```python
from build123d import *

# Parameters (mm, degrees)
BOSS_EXTRUDE1_DEPTH = 6
SKETCH2_R           = 5.25
CUT_EXTRUDE1_DEPTH  = 88
SKETCH2_2_R         = 5.25
BOSS_EXTRUDE2_DEPTH = 12
BOSS_EXTRUDE3_START = -24.75
SKETCH2_3_R         = 5.25
BOSS_EXTRUDE3_DEPTH = 10.25
SKETCH3_W           = 4
SKETCH3_H           = 8.859259966
BOSS_EXTRUDE4_DEPTH = 3
BOSS_EXTRUDE5_DEPTH = 3.5
CUT_EXTRUDE2_DEPTH  = 84.5
SKETCH14_W          = 24
SKETCH14_H          = 3
BOSS_EXTRUDE9_DEPTH = 0.5
BOSS_EXTRUDE7_DEPTH = 3.5
SKETCH12_W          = 11
SKETCH12_H          = 7.5
BOSS_EXTRUDE8_DEPTH = 8
SKETCH13_W          = 3
SKETCH13_H          = 5.5
CUT_EXTRUDE5_DEPTH  = 5.5
FILLET6_R           = 4.5
HOLE1_START         = -35
HOLE1_OUTLINE_R     = 3
HOLE1_DEPTH         = 70
CUT_EXTRUDE3_DEPTH  = 84.5
CHAMFER1_SIZE       = 2
FILLET3_R           = 2
BOSS_EXTRUDE6_REACH = 58.524
SKETCH9_W           = 1.5
SKETCH9_H           = 4
FILLET4_R           = 0.75
FILLET5_R           = 6


# Read off the part's stored shape, not the designer's step: Hole1
with BuildPart() as part:
    # Sketch1 → Boss-Extrude1 (new body)
    with BuildSketch(Plane.XY):
        Polygon((-25, 0), (25, 0), (35, 7.002075382), (35, 25), (-35, 25), (-35, 7.002075382), align=None)
    extrude(amount=BOSS_EXTRUDE1_DEPTH)

    # Sketch2 → Cut-Extrude1 (cut)
    with BuildSketch(Plane(origin=(35, 0, 0), x_dir=(0, 0, -1), z_dir=(1, 0, 0))):
        with Locations((-6, 12.452075382)):
            Circle(SKETCH2_R)
    extrude(amount=-CUT_EXTRUDE1_DEPTH, mode=Mode.SUBTRACT)

    # Sketch2<2> → Boss-Extrude2 (add)
    with BuildSketch(Plane(origin=(35, 0, 0), x_dir=(0, 0, -1), z_dir=(1, 0, 0))):
        with Locations((-6, 12.452075382)):
            Circle(SKETCH2_2_R)
    boss_extrude2 = extrude(amount=-BOSS_EXTRUDE2_DEPTH)

    # Sketch2<3> → Boss-Extrude3 (add)
    with BuildSketch(Plane(origin=(35, 0, 0), x_dir=(0, 0, -1), z_dir=(1, 0, 0)).offset(BOSS_EXTRUDE3_START)):
        with Locations((-6, 12.452075382)):
            Circle(SKETCH2_3_R)
    boss_extrude3 = extrude(amount=-BOSS_EXTRUDE3_DEPTH)

    # Sketch3 → Boss-Extrude4 (add)
    with BuildSketch(Plane(origin=(0, 0, 0), x_dir=(-1, 0, 0), z_dir=(0, 0, -1))):
        with Locations((2, -11.570370017)):
            Rectangle(SKETCH3_W, SKETCH3_H)
        Polygon((0, -7.140740034), (4, -7.140740034), (9, 0), (0, 0), align=None)
    boss_extrude4 = extrude(amount=-BOSS_EXTRUDE4_DEPTH)

    # Sketch4 → Boss-Extrude5 (add)
    with BuildSketch(Plane.XY.offset(6)):
        with BuildLine():
            Line((26, 10.749226565), (26, 18.202075382))
            ThreePointArc((26, 18.202075382), (28, 20.202075382), (30, 18.202075382))
            Line((30, 18.202075382), (30, 10.749226565))
            ThreePointArc((30, 10.749226565), (28, 8.749226565), (26, 10.749226565))
        make_face()
    boss_extrude5 = extrude(amount=BOSS_EXTRUDE5_DEPTH)

    # Sketch5 → Cut-Extrude2 (cut)
    with BuildSketch(Plane(origin=(35, 0, 0), x_dir=(0, 0, -1), z_dir=(1, 0, 0))):
        Polygon((-1, 25), (-1, 24.5), (-5, 21.5), (-5, 21), (-6, 21), (-6, 25), align=None)
    extrude(amount=-CUT_EXTRUDE2_DEPTH, mode=Mode.SUBTRACT)

    # Mirror2: Boss-Extrude2, Boss-Extrude3, Boss-Extrude4, Boss-Extrude5 across plane
    add(boss_extrude2.mirror(Plane(origin=(0, 0, 3), x_dir=(0, 0, 1), z_dir=(-1, 0, 0))))
    add(boss_extrude3.mirror(Plane(origin=(0, 0, 3), x_dir=(0, 0, 1), z_dir=(-1, 0, 0))))
    add(boss_extrude4.mirror(Plane(origin=(0, 0, 3), x_dir=(0, 0, 1), z_dir=(-1, 0, 0))))
    add(boss_extrude5.mirror(Plane(origin=(0, 0, 3), x_dir=(0, 0, 1), z_dir=(-1, 0, 0))))

    # Sketch14 → Boss-Extrude9 (add)
    with BuildSketch(Plane.XZ):
        with Locations((0, 4.5)):
            Rectangle(SKETCH14_W, SKETCH14_H)
    extrude(amount=BOSS_EXTRUDE9_DEPTH)

    # Sketch10 → Boss-Extrude7 (add)
    with BuildSketch(Plane.XY.offset(6)):
        with BuildLine():
            Line((-2, 12.452075382), (-2, 18.202075382))
            ThreePointArc((-2, 18.202075382), (0, 20.202075382), (2, 18.202075382))
            Line((2, 18.202075382), (2, 12.452075382))
            ThreePointArc((2, 12.452075382), (0, 10.452075382), (-2, 12.452075382))
        make_face()
    extrude(amount=BOSS_EXTRUDE7_DEPTH)

    # Sketch12 → Boss-Extrude8 (add, symmetric)
    with BuildSketch(Plane(origin=(0, 0, 0), x_dir=(0, 0, -1), z_dir=(1, 0, 0))):
        with Locations((-11.5, 14.25)):
            Rectangle(SKETCH12_W, SKETCH12_H)
    extrude(amount=BOSS_EXTRUDE8_DEPTH, both=True)

    # Sketch13 → Cut-Extrude5 (cut, symmetric)
    with BuildSketch(Plane(origin=(0, 0, 0), x_dir=(0, 0, -1), z_dir=(1, 0, 0))):
        with Locations((-13.5, 13.25)):
            Rectangle(SKETCH13_W, SKETCH13_H)
    extrude(amount=CUT_EXTRUDE5_DEPTH, both=True, mode=Mode.SUBTRACT)

    # Fillet6
    fillet6_edges = [part.edges().sort_by_distance(p)[0] for p in [
        (0, 18, 17),
    ]]
    fillet(fillet6_edges, radius=FILLET6_R)

    # Hole1 outline → Hole1 (cut)
    with BuildSketch(Plane.YZ.offset(HOLE1_START)):
        with Locations((12.452075382, 6)):
            Circle(HOLE1_OUTLINE_R)
    extrude(amount=HOLE1_DEPTH, mode=Mode.SUBTRACT)

    # Sketch7 → Cut-Extrude3 (cut)
    with BuildSketch(Plane.XY.offset(6)):
        with BuildLine():
            Line((-2.25, -1.75), (-2.25, 2.75))
            ThreePointArc((-2.25, 2.75), (0, 5), (2.25, 2.75))
            Line((2.25, 2.75), (2.25, -1.75))
            ThreePointArc((2.25, -1.75), (0, -4), (-2.25, -1.75))
        make_face()
    extrude(amount=-CUT_EXTRUDE3_DEPTH, mode=Mode.SUBTRACT)

    # Chamfer1
    chamfer1_edges = [part.edges().sort_by_distance(p)[0] for p in [
        (0, 5, 0),
        (0, -4, 0),
        (-2.25, 0.5, 0),
        (2.25, 0.5, 0),
    ]]
    chamfer(chamfer1_edges, length=CHAMFER1_SIZE)

    # Fillet3
    fillet3_edges = [part.edges().sort_by_distance(p)[0] for p in [
        (-35, 25, 0.5),
        (35, 25, 0.5),
    ]]
    fillet(fillet3_edges, radius=FILLET3_R)

    # Boss-Extrude6: up to this face of the body (flat: up to its plane)
    boss_extrude6_end = Plane(part.part.faces().sort_by_distance((0, 22.996608877, 3.004521497))[0])
    # Sketch9 → Boss-Extrude6 (add, up to the picked face)
    with BuildSketch(Plane(origin=(0, 25, 0), x_dir=(1, 0, 0), z_dir=(0, 1, 0)), mode=Mode.PRIVATE) as boss_extrude6_sk1:
        with Locations((0, -2)):
            Rectangle(SKETCH9_W, SKETCH9_H)
    boss_extrude6_tool1 = split(extrude(boss_extrude6_sk1.sketch, amount=-BOSS_EXTRUDE6_REACH, mode=Mode.PRIVATE), bisect_by=boss_extrude6_end, keep=Keep.BOTH, mode=Mode.PRIVATE)
    # Sketch9 → Boss-Extrude6 (add, up to the picked face)
    with BuildSketch(Plane(origin=(0, 25, 0), x_dir=(1, 0, 0), z_dir=(0, 1, 0)), mode=Mode.PRIVATE) as boss_extrude6_sk2:
        with Locations((-6, -2)):
            Rectangle(SKETCH9_W, SKETCH9_H)
    boss_extrude6_tool2 = split(extrude(boss_extrude6_sk2.sketch, amount=-BOSS_EXTRUDE6_REACH, mode=Mode.PRIVATE), bisect_by=boss_extrude6_end, keep=Keep.BOTH, mode=Mode.PRIVATE)
    add(boss_extrude6_tool1.solids().sort_by(Axis((0, 25, 2), (0, -1, 0)))[0])
    add(boss_extrude6_tool2.solids().sort_by(Axis((-6, 25, 2), (0, -1, 0)))[0])

    # Fillet4
    fillet4_edges = [part.edges().sort_by_distance(p)[0] for p in [
        (-6.75, 23.625, 4),
        (-5.25, 23.625, 4),
        (-0.75, 23.625, 4),
        (0.75, 23.625, 4),
    ]]
    fillet(fillet4_edges, radius=FILLET4_R - 0.0001)  # a hair under: the kernel refuses the full size

    # Fillet5
    fillet5_edges = [part.edges().sort_by_distance(p)[0] for p in [
        (4, -7.140740034, 1.5),
        (-4, -7.140740034, 1.5),
    ]]
    fillet(fillet5_edges, radius=FILLET5_R)


solid = part.part
```
The model under review builds one solid part; all positions refer to its coordinate system, in mm. A direction names the side the tool comes from. Give positions to 0.01 mm unless a question says otherwise; leave off trailing zeros. Loops run counter-clockwise (first coordinate to the right, second up) from the corner with the lowest first, then second, coordinate; pieces in that order, holes last. Notation, with made-up numbers: (86, 30) - (131, 30) arc R16 cw to (131, 57) - close; hole circle Ø10 at (6.25, -25.75). An arc over 180 degrees is marked (long way). Answer as a JSON object with one key per item and string values.
Q1. Mouldability with a two-part tool opening along Y and no side actions: class faces 5 (the conical face through (-0.1, -4.3, 1.7)), 6 (the flat face through (7.02, -2.83, 1.48)), 7 (the flat face through (4, -13, 1)) as +Y half, -Y half, draft (parallel to the pull), parting line (faces both ways), or undercut.
Worked out:
{"face 5": "undercut", "face 6": "-Y half", "face 7": "draft"}
Q2. Insertion check: pin 1 (1.9 mm diameter, centred on x = -28.5, y = 19, fed in from +Z); pin 2 (1.2 mm diameter, centred on y = -0.5, z = 4, fed in from +X); pin 3 (2 mm diameter, centred on y = 1.5, z = 4, fed in from -X); pin 4 (3 mm diameter, centred on y = -3.5, z = 5, fed in from -X). Each pin has a flat end and moves straight along its axis. Give the tip position at first contact, or say it passes through.
Worked out:
{"pin 1": "stops at z = 9.5", "pin 2": "stops at x = 25.14", "pin 3": "stops at x = -28.57", "pin 4": "passes through"}
Q3. Add section A-A on x = -28. State the section outline as (y, z) points.
Worked out:
{"outline": "(2.1, 0) - (25, 0) - (25, 1) - (24.5, 1) - (21.5, 5) - (21, 5) - (21, 6) - (20.2, 6) - (20.2, 9.5) - (16.37, 9.5) arc R5.25 ccw to (7.2, 6) - (2.1, 6) - close; hole circle Ø6 at (12.45, 6)"}
Q4. To check wall thickness, follow line 1 along Z through (x, y) = (-4, 12); line 2 along Y through (x, z) = (0.5, 5.25); line 3 along Y through (x, z) = (6, 8). State the ranges of each line that lie inside material, in increasing order.
Worked out:
{"line 1": "z = 0 to 3.03, 8.97 to 12, 15 to 17", "line 2": "y = 4.94 to 9.55, 15.36 to 21", "line 3": "y = 7.6 to 10.22, 14.69 to 18"}
Q5. For faces 1 (the flat face through (30, 18, 8)), 2 (the flat face through (-4, -13, 1)), 3 (the flat face through (-2.25, 1, 4)), 4 (the cylindrical face through (-16.54, 12.34, 0.75)), list the 3-axis set-ups (+Z, -Z, +X, -X, +Y, -Y) from which the entire face can be reached by the end or side of a thin tool; tool diameter is ignored.
Worked out:
{"face 1": "+Z, +X, +Y", "face 2": "+Z, -Z, -X, -Y", "face 3": "+Z, -Z", "face 4": "+Z"}
Q6. Add section B-B on x = -20. State the section outline as (y, z) points, plus the area to 3 significant figures.
Worked out:
{"outline": "(0, 0) - (25, 0) - (25, 1) - (24.5, 1) - (21.5, 5) - (21, 5) - (21, 6) - (17.7, 6) arc R5.25 cw to (7.2, 6) - (0, 6) - close", "area": "94.7 mm^2"}
Q7. Add section C-C on x = 29. State the section outline as (y, z) points, plus the area to 3 significant figures.
Worked out:
{"outline": "(2.8, 0) - (25, 0) - (25, 1) - (24.5, 1) - (21.5, 5) - (21, 5) - (21, 6) - (19.93, 6) - (19.93, 9.5) - (16.37, 9.5) arc R5.25 ccw to (7.2, 6) - (2.8, 6) - close; hole circle Ø6 at (12.45, 6)", "area": "145 mm^2"}
